CAD build for the part. Positions are in the model's coordinates, mm. A direction names the side the tool comes from. Coordinates: 2 decimals unless noted, no trailing zeros. Loops run counter-clockwise (first coordinate to the right, second up) from the corner with the lowest first, then second, coordinate; pieces in that order, holes last. Notation, with made-up numbers: (-16, -2) -> (25, -2) arc R31 ccw to (25, 37) -> close; hole circle Ø10 at (2.25, 58). An arc over 180 degrees is marked (long way). Write item = value, one per line. Start each with the question number.
(1) Band-saw the part on D-D (z = 3). Write the cut outline in (x, y).
(2) Band-saw the part on B-B (z = -0.5). Write the cut outline in (x, y), and give its area (3 significant figures).
(3) Flat gauge pins, fed straight in: P1, Ø2, axis at y = 1, z = -1.5, coming from the +X side; P2, Ø1, axis at y = 1, z = 3, coming from the +X side; P3, Ø3, axis at x = 1.5, y = -1.5, coming from the +Z side. Where does each tip first touch, or does it go through?
(4) Band-saw the part on C-C (y = -1.1). Write the cut outline in (x, z) (3 decimals).
(5) Band-saw the part on A-A (x = 0). Write the cut outline in (y, z), and give its area (3 significant figures).
(6) Tool access for faces 1 (the face through (0.54, -2.44, 3.56)), 2 (the face through (2.5, 0, 0.5)): list every direction of +Z, -Z, +X, -X, +Y, -Y with a clear straight run to the whole face (end or side of a thin tool).
(7) Drill centre lines: line 1 (X direction, y = 0.05, z = 3.5); line 2 (Z direction, x = -1.85, y = 2.1); line 3 (Z direction, x = 1.85, y = 1.05). Where is each one in solid material? Low to high. Write a range as from..to.
Autodesk Fusion 360 part; units mm, degrees
sketch "スケッチ1" plane through (0, 0, 0) normal (0, 0, 1) x (1, 0, 0)
  circle A0 centre (0, 0) radius 2.9
  line L0 (2.5, 1.4697) -> (2.5, -1.4697)
  circle A1 centre (-1.27, 0) radius 0.25
  line L1 (-3.5255, 0) -> (3.8644, 0) construction
  line L2 (0, 3.5138) -> (0, -4.0944) construction
  circle A2 centre (1.27, 0) radius 0.25
  dimension "d1" = 5.8
  dimension "d8" = 2.5
  dimension "d11" = 0.5
  dimension "d14" = 1.27
extrude "押し出し1" add sketch "スケッチ1" along normal blind 1 contours A0 L0 | A0 L0 | A1 | A2
sketch "スケッチ2" plane through (0, 0, 1) normal (0, 0, 1) x (-1, 0, 0)
  circle A0 centre (0, 0) radius 2.9
  circle A1 centre (0, 0) radius 2.5
  dimension "d4" = 5
extrude "押し出し2" add sketch "スケッチ2" along normal blind 7.7 contours A1
fillet "フィレット1" radius 2.5 1 edges at (2.3308, 0.904, 8.7)
extrude "押し出し3" cut sketch "スケッチ1" along normal blind 1 contours A0 L0 picked at (2.5576, -0.3752)
extrude "押し出し4" add sketch "スケッチ1" against normal blind 5 contours A1
extrude "押し出し5" add sketch "スケッチ1" against normal blind 3.5 contours A2
Findings below:
q1.outline = circle Ø5 at (0, 0)
q2.outline = circle Ø0.5 at (-1.27, 0); circle Ø0.5 at (1.27, 0)
q2.area = 0.393 mm²
q3.P1 = 1.52
q3.P2 = 2.45
q3.P3 = 8.62
q4.outline = (-2.683, 0) -> (2.5, 0) -> (2.5, 1) -> (2.245, 1) -> (2.245, 6.2) arc R2.245 ccw to (-2.245, 6.2) -> (-2.245, 1) -> (-2.683, 1) -> close
q5.outline = (-2.9, 0) -> (2.9, 0) -> (2.9, 1) -> (2.5, 1) -> (2.5, 6.2) arc R2.5 ccw to (-2.5, 6.2) -> (-2.5, 1) -> (-2.9, 1) -> close
q5.area = 41.6 mm²
q6.face_1 = +Z
q6.face_2 = +Z, -Z, +X, +Y, -Y
q7.line_1 = -2.5..2.5
q7.line_2 = 0..1
q7.line_3 = 0..7.51
